Work out the finished part from the listing and answer in its coordinate system (mm). Face numbers are marked on the shaded views. A direction names the side the tool comes from. Round coordinates to 2 decimals unless told otherwise and drop trailing zeros. Write each loop counter-clockwise with the first axis right and the second up, starting at its lowest first coordinate (ties: lowest second). Pieces come first, ordered by that corner, then holes. Notation, with made-up numbers: (70.5, 63) -> (110.5, 63) arc R17 ccw to (110.5, 76) -> close; hole circle Ø5 at (-28.75, 29.25). An arc over 180 degrees is marked (long way). One line per question, with ' | ' between items. Start each with the question number.
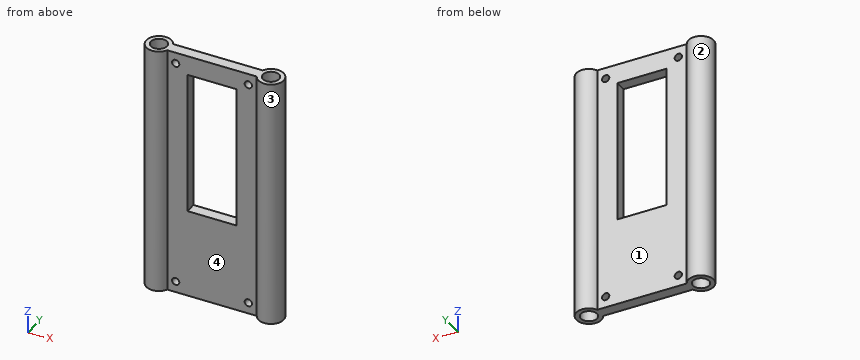
```python
from build123d import *

# Parameters (mm, degrees)
SKETCH1_R           = 3.683
BOSS_EXTRUDE1_DEPTH = 114.3
SKETCH2_R           = 1.651
SKETCH2_W           = 22.225
SKETCH2_H           = 65.0875
CUT_EXTRUDE1_DEPTH  = 114.3


with BuildPart() as part:
    # Sketch1 → Boss-Extrude1 (new body)
    with BuildSketch(Plane.XY):
        with BuildLine():
            ThreePointArc((-20.28046633, 2.54), (-31.115, 0), (-20.28046633, -2.54))
            Line((-20.28046633, -2.54), (20.28046633, -2.54))
            ThreePointArc((20.28046633, -2.54), (31.115, 0), (20.28046633, 2.54))
            Line((20.28046633, 2.54), (-20.28046633, 2.54))
        make_face()
        with Locations((-25.4, 0)):
            Circle(SKETCH1_R, mode=Mode.SUBTRACT)
        with Locations((25.4, 0)):
            Circle(SKETCH1_R, mode=Mode.SUBTRACT)
    extrude(amount=-BOSS_EXTRUDE1_DEPTH)

    # Sketch2 → Cut-Extrude1 (cut)
    with BuildSketch(Plane(origin=(0, 2.54, 0), x_dir=(1, 0, 0), z_dir=(0, 1, 0))):
        with Locations(Location((-16.47046633, 109.22, 0), (0, 0, 270))):
            Circle(SKETCH2_R)
        with Locations(Location((16.47046633, 109.22, 0), (0, 0, 270))):
            Circle(SKETCH2_R)
        with Locations(Location((-16.47046633, 5.08, 0), (0, 0, 270))):
            Circle(SKETCH2_R)
        with Locations(Location((16.47046633, 5.08, 0), (0, 0, 270))):
            Circle(SKETCH2_R)
        with Locations((0, 41.43375)):
            Rectangle(SKETCH2_W, SKETCH2_H)
    extrude(amount=-CUT_EXTRUDE1_DEPTH, mode=Mode.SUBTRACT)


solid = part.part
```
(1) A cutting plane is placed at B-B, the plane z = -109.22. Determine the outline of the cut face in (x, y) (3 decimals), then the cut area to 3 significant figures.
(2) For the marked faces 1 and 2, determine the directions among +Z, -Z, +X, -X, +Y, -Y from which every point of the face is accessible in a straight line to the end or side of a thin tool.
(3) A cutting plane is placed at D-D, the plane z = -76. Determine the outline of the cut face in (x, y) (3 decimals).
(4) Consider L1, parallel to X at y = -0.25, z = -103.5; L2, parallel to X at y = 0.4, z = -5.08; L3, parallel to Z at x = 5.5, y = 2.5. Determine where each line is inside the solid, lowest interval first.
(5) The mould has two halves that part along X. Classify the marked faces 3 and 4: +X half, -X half, draft (parallel to the pull), parting line (faces both ways), or undercut.
(6) A cutting plane is placed at A-A, the plane z = -55. Determine the outline of the cut face in (x, y) (1 decimal).
(7) A cutting plane is placed at C-C, the plane x = 5. Determine the outline of the cut face in (y, z).
(8) Given pin 1 Ø4 at (x, z) = (-16.47, -109.22) entering from +Y; pin 2 Ø12 at (x, z) = (7, -90.5) entering from -Y, each flat-ended and moving along its own axis, determine where each tip first touches the part or whether it passes through.
Returned:
1) outline: (-20.28, -2.54) -> (-18.121, -2.54) -> (-18.121, 2.54) -> (-20.28, 2.54) arc R5.715 ccw (long way) to start; (-14.819, -2.54) -> (14.819, -2.54) -> (14.819, 2.54) -> (-14.819, 2.54) -> close; (18.121, -2.54) -> (20.28, -2.54) arc R5.715 ccw (long way) to (20.28, 2.54) -> (18.121, 2.54) -> close; hole circle Ø7.366 at (-25.4, 0); hole circle Ø7.366 at (25.4, 0) | area: 288 mm2
2) face 1: +Z, -Z, +Y | face 2: +Z, -Z
3) outline: (-20.28, -2.54) -> (20.28, -2.54) arc R5.715 ccw (long way) to (20.28, 2.54) -> (-20.28, 2.54) arc R5.715 ccw (long way) to start; hole circle Ø7.366 at (-25.4, 0); hole circle Ø7.366 at (25.4, 0)
4) L1: -31.11 to -29.07, -21.73 to 21.73, 29.07 to 31.11 | L2: -31.1 to -29.06, -21.74 to -18.12, -14.82 to 14.82, 18.12 to 21.74, 29.06 to 31.1 | L3: -114.3 to -73.98, -8.89 to 0
5) face 3: undercut | face 4: undercut
6) outline: (-20.3, -2.5) -> (-11.1, -2.5) -> (-11.1, 2.5) -> (-20.3, 2.5) arc R5.7 ccw (long way) to start; (11.1, -2.5) -> (20.3, -2.5) arc R5.7 ccw (long way) to (20.3, 2.5) -> (11.1, 2.5) -> close; hole circle Ø7.4 at (-25.4, 0); hole circle Ø7.4 at (25.4, 0)
7) outline: (-2.54, -114.3) -> (2.54, -114.3) -> (2.54, -73.98) -> (-2.54, -73.98) -> close; (-2.54, -8.89) -> (2.54, -8.89) -> (2.54, 0) -> (-2.54, 0) -> close
8) pin 1: y = 2.54 | pin 2: y = -2.54
